Could you check a few things on this model? Use its own coordinates, in mm. A direction names the side the tool comes from. Give positions to 0.01 mm unless a question says otherwise; leave off trailing zeros. Write each loop counter-clockwise with the first axis right and the second up, starting at its lowest first coordinate (ties: lowest second). Pieces come first, ordered by that corner, then holes. Notation, with made-up numbers: (40.5, 80.5) - (98.5, 80.5) arc R19 ccw to (98.5, 95.5) - close; hole circle Ø2 at (-36.5, 83.25). An arc over 180 degrees is marked (long way). Answer as CSV lines item,"result". Start each with the question number.
Q1. Imagine slicing it at B-B on z = -29. List the corners of the cut face in (x, y) for me, and give its area (3 significant figures).
Q2. On a 3-axis mill with a long thin cutter (end or side, diameter ignored), from which of +Z, -Z, +X, -X, +Y, -Y can I reach the whole of each face in a straight line? I mean faces 4 (the face through (0, -576, -60)), 5 (the face through (457, -100, -60)), 6 (the face through (225, -30, -60)). Say none if no direction works.
Q3. Will these pins go through, and if not, where does the flat tip stop? pin 1 Ø3 at (y, z) = (-545.5, -48.5) entering from -X; pin 2 Ø6.5 at (x, y) = (10.5, -4) entering from +Z; pin 3 Ø1.2 at (x, z) = (-188, -68) entering from -Y.
Q4. If I drill on line 1 along X through (y, z) = (-482, -52); line 2 along X through (y, z) = (-487, -5); line 3 along Y through (x, z) = (367, -60.5), over which ranges is the centre line in solid material (lowest first)?
Q5. We'd pull the mould along X, two halves only. Please class faces 1 (the face through (0, -100, -60)), 2 (the face through (-415, -345, -30)), 3 (the face through (-230, -650, -60)): pulls with the +X half, pulls with the -X half, needs draft (parallel to the pull), parting line crosses it, or undercut.
Q6. Imagine slicing it at A-A on y = -445. List the corners of the cut face in (x, z) for me, and give its area (3 significant figures).
Q7. Imagine slicing it at C-C on x = -254. List the corners of the cut face in (y, z) for me.
```python
from build123d import *

# Parameters (mm, degrees)
SKETCH1_W           = 990
SKETCH1_H           = 680
BOSS_EXTRUDE1_DEPTH = 70
SKETCH2_W           = 990
SKETCH2_H           = 379
CUT_EXTRUDE1_DEPTH  = 10
CUT_EXTRUDE2_DEPTH  = 1204.079382252
CUT_EXTRUDE4_DEPTH  = 844.993483387


with BuildPart() as part:
    # Sketch1 → Boss-Extrude1 (new body)
    with BuildSketch(Plane.XY):
        with Locations((0, -340)):
            Rectangle(SKETCH1_W, SKETCH1_H)
    extrude(amount=-BOSS_EXTRUDE1_DEPTH)

    # Sketch2 → Cut-Extrude1 (cut)
    with BuildSketch(Plane(origin=(0, 0, -70), x_dir=(-1, 0, 0), z_dir=(0, 0, -1))):
        with Locations((0, -334.5)):
            Rectangle(SKETCH2_W, SKETCH2_H)
    extrude(amount=-CUT_EXTRUDE1_DEPTH, mode=Mode.SUBTRACT)

    # Sketch3 → Cut-Extrude2 (cut, through all)
    with BuildSketch(Plane.ZY.offset(495)):
        with BuildLine():
            Line((-134, -680), (-66, -680))
            ThreePointArc((-66, -680), (-61.757359313, -678.242640687), (-60, -674))
            Line((-60, -674), (-60, -626))
            ThreePointArc((-60, -626), (-61.757359313, -621.757359313), (-66, -620))
            Line((-66, -620), (-134, -620))
            ThreePointArc((-134, -620), (-138.242640687, -621.757359313), (-140, -626))
            Line((-140, -626), (-140, -674))
            ThreePointArc((-140, -674), (-138.242640687, -678.242640687), (-134, -680))
        make_face()
        with BuildLine():
            Line((-134, -60), (-66, -60))
            ThreePointArc((-66, -60), (-61.757359313, -58.242640687), (-60, -54))
            Line((-60, -54), (-60, -6))
            ThreePointArc((-60, -6), (-61.757359313, -1.757359313), (-66, 0))
            Line((-66, 0), (-134, 0))
            ThreePointArc((-134, 0), (-138.242640687, -1.757359313), (-140, -6))
            Line((-140, -6), (-140, -54))
            ThreePointArc((-140, -54), (-138.242640687, -58.242640687), (-134, -60))
        make_face()
    extrude(amount=-CUT_EXTRUDE2_DEPTH, mode=Mode.SUBTRACT)

    # Sketch5 → Cut-Extrude4 (cut, through all)
    with BuildSketch(Plane.XZ.offset(680)):
        with BuildLine():
            ThreePointArc((495, -6), (493.242640687, -1.757359313), (489, 0))
            Line((489, 0), (489, -60))
            ThreePointArc((489, -60), (493.242640687, -58.242640687), (495, -54))
            Line((495, -54), (495, -6))
        make_face()
        with BuildLine():
            Line((489, 0), (421, 0))
            ThreePointArc((421, 0), (416.757359313, -1.757359313), (415, -6))
            Line((415, -6), (415, -54))
            ThreePointArc((415, -54), (416.757359313, -58.242640687), (421, -60))
            Line((421, -60), (489, -60))
            Line((489, -60), (489, 0))
        make_face()
        with BuildLine():
            Line((34, 0), (-34, 0))
            ThreePointArc((-34, 0), (-38.242640687, -1.757359313), (-40, -6))
            Line((-40, -6), (-40, -54))
            ThreePointArc((-40, -54), (-38.242640687, -58.242640687), (-34, -60))
            Line((-34, -60), (34, -60))
            ThreePointArc((34, -60), (38.242640687, -58.242640687), (40, -54))
            Line((40, -54), (40, -6))
            ThreePointArc((40, -6), (38.242640687, -1.757359313), (34, 0))
        make_face()
        with BuildLine():
            Line((-489, 0), (-489, -60))
            Line((-489, -60), (-421, -60))
            ThreePointArc((-421, -60), (-416.757359313, -58.242640687), (-415, -54))
            Line((-415, -54), (-415, -6))
            ThreePointArc((-415, -6), (-416.757359313, -1.757359313), (-421, 0))
            Line((-421, 0), (-489, 0))
        make_face()
        with BuildLine():
            ThreePointArc((-495, -54), (-493.242640687, -58.242640687), (-489, -60))
            Line((-489, -60), (-489, 0))
            ThreePointArc((-489, 0), (-493.242640687, -1.757359313), (-495, -6))
            Line((-495, -6), (-495, -54))
        make_face()
        with BuildLine():
            Line((-495, -60), (-489, -60))
            ThreePointArc((-489, -60), (-493.242640687, -58.242640687), (-495, -54))
            Line((-495, -54), (-495, -60))
        make_face()
        with BuildLine():
            ThreePointArc((-495, -6), (-493.242640687, -1.757359313), (-489, 0))
            Line((-489, 0), (-495, 0))
            Line((-495, 0), (-495, -6))
        make_face()
        with BuildLine():
            Line((495, 0), (489, 0))
            ThreePointArc((489, 0), (493.242640687, -1.757359313), (495, -6))
            Line((495, -6), (495, 0))
        make_face()
        with BuildLine():
            ThreePointArc((495, -54), (493.242640687, -58.242640687), (489, -60))
            Line((489, -60), (495, -60))
            Line((495, -60), (495, -54))
        make_face()
    extrude(amount=-CUT_EXTRUDE4_DEPTH, mode=Mode.SUBTRACT)


solid = part.part
```
Conclusion:
1,outline,"(-415, -680) - (-40, -680) - (-40, 0) - (-415, 0) - close; (40, -680) - (415, -680) - (415, 0) - (40, 0) - close"
1,area,"510,000 mm^2"
2,face 4,"+Z, +Y, -Y"
2,face 5,"+Z, +X, +Y, -Y"
2,face 6,"-Z, +X, -X"
3,pin 1,"x = -415"
3,pin 2,"z = -60"
3,pin 3,"y = -620"
4,line 1,"-415 to -40, 40 to 415"
4,line 2,"-415.08 to -39.92, 39.92 to 415.08"
4,line 3,"-680 to -676.4, -623.6 to -524, -145 to -56.4, -3.6 to 0"
5,face 1,"undercut"
5,face 2,"pulls with the -X half"
5,face 3,"needs draft"
6,outline,"(-421, -60) - (-34, -60) arc R6 cw to (-40, -54) - (-40, -6) arc R6 cw to (-34, 0) - (-421, 0) arc R6 cw to (-415, -6) - (-415, -54) arc R6 cw to start; (34, -60) - (421, -60) arc R6 cw to (415, -54) - (415, -6) arc R6 cw to (421, 0) - (34, 0) arc R6 cw to (40, -6) - (40, -54) arc R6 cw to start"
6,area,"45,100 mm^2"
7,outline,"(-680, -66) arc R6 cw to (-674, -60) - (-626, -60) arc R6 cw to (-620, -66) - (-620, -70) - (-524, -70) - (-524, -60) - (-145, -60) - (-145, -70) - (-60, -70) - (-60, -66) arc R6 cw to (-54, -60) - (-6, -60) arc R6 cw to (0, -66) - (0, 0) - (-680, 0) - close"
